Study the drawing (mm; zero at the part's minimum x, y, z) and answer. Coordinates: 2 decimals unless noted, no trailing zeros. Loops run counter-clockwise (first coordinate to the right, second up) from the corner with the lowest first, then second, coordinate; pieces in that order, holes last. Notation, with made-up numbers: (63.25, -6) -> (106.25, -6) arc R32 ccw to (106.25, 33) -> close; hole circle Ø4 at (23.5, 24). An arc over 180 degrees is marked (long way). Answer in a Markdown table with one row per item.
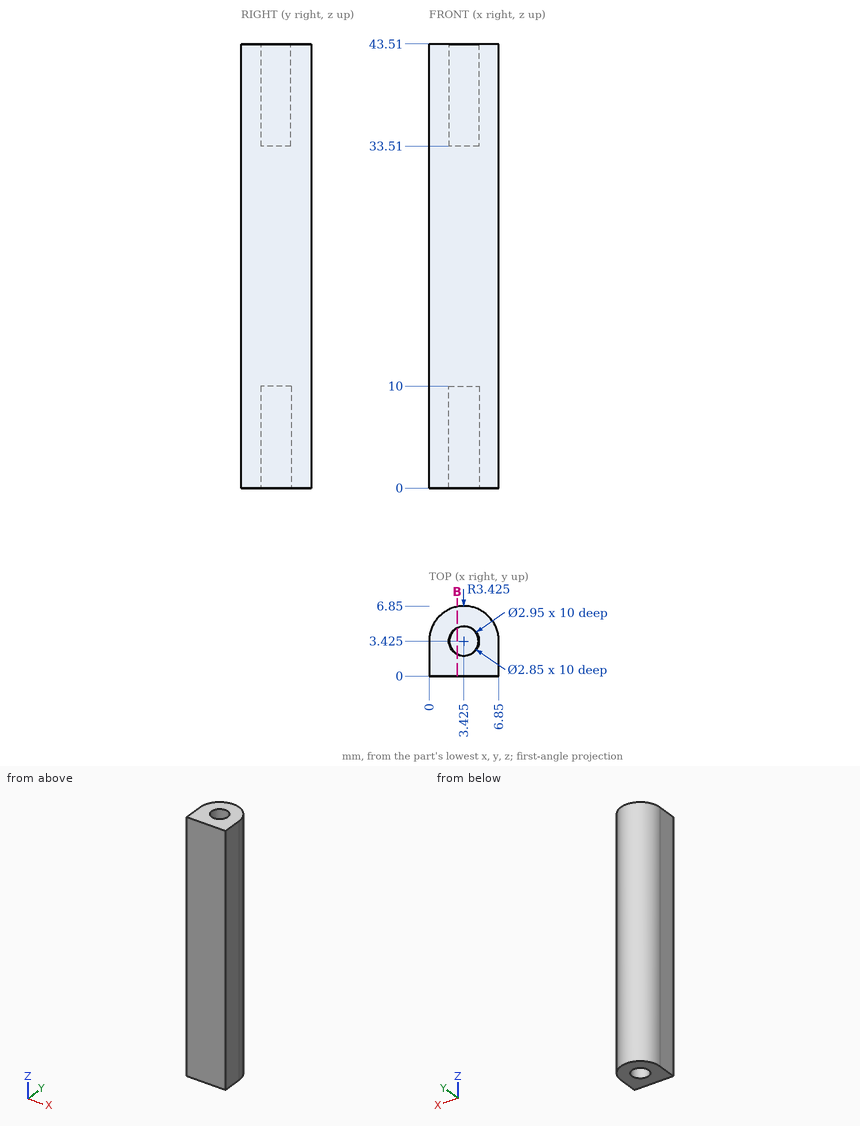
1. Given pin 1 Ø1.7 at (x, y) = (3.425, 3.425) entering from +Z; pin 2 Ø1 at (y, z) = (4.5, 28) entering from +X; pin 3 Ø1.5 at (x, z) = (0.5, 14.5) entering from +Y, each flat-ended and moving along its own axis, determine where each tip first touches the part or whether it passes through.
A:
| item | result |
|---|---|
| pin 1 | stops at z = 33.51 |
| pin 2 | stops at x = 6.8 |
| pin 3 | stops at y = 6.07 |
2. A cutting plane is placed at B-B on x = 2.75. Give the vertices of the cut face in (y, z).
A:
| item | result |
|---|---|
| outline | (0, 0) -> (2.11, 0) -> (2.11, 10) -> (4.74, 10) -> (4.74, 0) -> (6.78, 0) -> (6.78, 43.51) -> (4.68, 43.51) -> (4.68, 33.51) -> (2.17, 33.51) -> (2.17, 43.51) -> (0, 43.51) -> close |
3. Find the intervals of material crossed by probe 1 along Z at (x, y) = (3.25, 4.75); probe 2 along Y at (x, z) = (3.5, 5.5); probe 3 along Y at (x, z) = (4.5, 40) (1 decimal), in increasing order.
A:
| item | result |
|---|---|
| probe 1 | z = 10 to 33.51 |
| probe 2 | y = 0 to 1.95, 4.9 to 6.85 |
| probe 3 | y = 0 to 2.5, 4.4 to 6.7 |
